Input: part model. Units: mm. Frame: model coordinates. A direction names the side the tool comes from. Give positions to 0.01 mm unless a question says otherwise; leave off trailing zeros. Order: outer loops, then holes, each group sorted by start corner. A loop starts at its lowest first (then second) coordinate and runs counter-clockwise, first axis right, second up.
```python
from build123d import *

# Parameters (mm, degrees)
SKETCH_1_R      = 6
EXTRUDE_1_DEPTH = 6
CHAMFER_1_SIZE  = 0.5


with BuildPart() as part:
    # Эскиз1 → Бобышка-Вытянуть1 (new, symmetric)
    with BuildSketch(Plane.XY):
        with BuildLine():
            Line((0, 24), (14, 10))
            Line((14, 10), (14, -16.411542732))
            Line((14, -16.411542732), (5, -50))
            Line((5, -50), (-5, -50))
            ThreePointArc((-5, -50), (-14.257815193, -43.780589618), (-12, -32.858571571))
            Line((-12, -32.858571571), (-12, -12.141428429))
            ThreePointArc((-12, -12.141428429), (-12.780455543, -8.268445082), (-15, -5))
            Line((-15, -5), (-15, 2.858571571))
            ThreePointArc((-15, 2.858571571), (-12.028827286, 9.241241333), (-14, 16))
            ThreePointArc((-14, 16), (-14.472135955, 21.236067977), (-10, 24))
            Line((-10, 24), (0, 24))
        make_face()
        Circle(SKETCH_1_R, mode=Mode.SUBTRACT)
    extrude(amount=EXTRUDE_1_DEPTH, both=True)

    # Фаска1
    chamfer_1_edges = [part.edges().sort_by_distance(p)[0] for p in [
        (-6, 0, -6),
        (-6, 0, 6),
    ]]
    chamfer(chamfer_1_edges, length=CHAMFER_1_SIZE)


solid = part.part
```
1) Pull-direction query (X, two-part tool) for faces 1 (the face through (-6, 0, 0)), 2 (the face through (-14.194, -43.933, 0.084)), 3 (the face through (0, -12, -6)); classes: pulls with the +X half, pulls with the -X half, needs draft (parallel to the pull), parting line crosses it, or undercut.
2) Cut plane A-A (y = 0). Return the cut outline in (x, z), then the cut area to 4 significant figures.
3) Cut plane B-B (z = 3.5). Return the cut outline in (x, y).
4) Line query: probe 1 along Y at (x, z) = (0, 1.5); probe 2 along X at (y, z) = (-1, 3.25); probe 3 along Y at (x, z) = (4, 3.75). Output: solid intervals per line, ascending.
5) Reachability of faces 4 (the face through (7, 17, 0)), 5 (the face through (-12.76, -8.32, 0.08)) from +Z, -Z, +X, -X, +Y, -Y: full face, straight path, thin tool, end or side. Return the list, or none.
6) First-contact query: P1, Ø4, axis at y = -33.5, z = -1, coming from the +X side; P2, Ø3.5, axis at y = -19.5, z = -2.5, coming from the -X side; P3, Ø4, axis at y = 6.5, z = -1.5, coming from the -X side. Flat tips, straight axial feed; report the tip coordinate or a pass-through.
7) Cut plane C-C (x = -13). Return the cut outline in (y, z).
8) Cut plane D-D (y = 19.5). Return the cut outline in (x, z), then the cut area to 3 significant figures.
Geometry says:
1. face 1: undercut
1. face 2: pulls with the -X half
1. face 3: needs draft
2. outline: (-15, -6) - (-6.5, -6) - (-6, -5.5) - (-6, 5.5) - (-6.5, 6) - (-15, 6) - close; (6, -5.5) - (6.5, -6) - (14, -6) - (14, 6) - (6.5, 6) - (6, 5.5) - close
2. area: 203.5 mm2
3. outline: (-15, -5) arc R10 cw to (-12, -12.14) - (-12, -32.86) arc R10 ccw to (-5, -50) - (5, -50) - (14, -16.41) - (14, 10) - (0, 24) - (-10, 24) arc R5 ccw to (-14, 16) arc R10 cw to (-15, 2.86) - close; hole circle Ø12 at (0, 0)
4. probe 1: y = -50 to -6, 6 to 24
4. probe 2: x = -15 to -5.92, 5.92 to 14
4. probe 3: y = -50 to -4.47, 4.47 to 20
5. face 4: +Z, -Z, +X, +Y
5. face 5: +Z, -Z, -X
6. P1: stops at x = 9.96
6. P2: stops at x = -12
6. P3: stops at x = -13.65
7. outline: (-46, -6) - (-34, -6) - (-34, 6) - (-46, 6) - close; (-7.78, -6) - (5.64, -6) - (5.64, 6) - (-7.78, 6) - close; (14.36, -6) - (23, -6) - (23, 6) - (14.36, 6) - close
8. outline: (-14.97, -6) - (4.5, -6) - (4.5, 6) - (-14.97, 6) - close
8. area: 234 mm2
